Check sheet for the modelled part. Datum: model origin and axes. Units: mm. A direction names the side the tool comes from. Give positions to 0.01 mm unless a question says otherwise; leave off trailing zeros. Order: outer loops, then holes, each group sorted by start corner. A loop starts at its lowest first (then second) coordinate and runs counter-clockwise, first axis right, second up. Notation, with made-up numbers: M -32,50.5 L 2,50.5 A11 cw 2,60.5 Z; hole C 67.25,9.5 d1. An arc over 180 degrees is marked long. Answer in a Markdown table with one row per item. Add a question column.
Autodesk Inventor part; units mm, degrees
ref_plane "YZ Plane" through (0, 0, 0) normal (1, 0, 0) x (0, 1, 0)
ref_plane "XZ Plane" through (0, 0, 0) normal (0, 1, 0) x (-1, 0, 0)
ref_plane "XY Plane" through (0, 0, 0) normal (0, 0, 1) x (1, 0, 0)
sketch "Sketch1" plane through (0, 0, 0) normal (0, 1, 0) x (-1, 0, 0)
  circle A0 centre (0, 0) radius 22.5
  circle A1 centre (0, 0) radius 19
  dimension "d0" = 45
  dimension "d1" = 38
extrude "Extrusion1" add sketch "Sketch1" along normal blind 10
sketch "Sketch2" plane through (0, 10, 0) normal (0, 1, 0) x (1, 0, 0)
  circle A0 centre (0, 0) radius 22.5
  line L0 (0, -22.5) -> (0, 22.5) construction
  circle A1 centre (0, 0) radius 19
  line L1 (-19, 0) -> (19, 0) construction
sketch "Sketch3" plane through (0, 10, 0) normal (0, 1, 0) x (1, 0, 0)
  line L0 (-8, -20) -> (8, -20)
  line L1 (8, -20) -> (8, -40)
  line L2 (8, -40) -> (-8, -40)
  line L3 (-8, -40) -> (-8, -20)
  point P0 (0, 0)
  dimension "d4" = 16
  dimension "d5" = 20
  dimension "d6" = 20
  dimension "d7" = 8
extrude "Extrusion2" add sketch "Sketch3" against normal blind 3
pattern_circular "Circular Pattern1" count 2 over 360 about axis through (0, 0, 0) along (0, 1, 0) of "Extrusion2"
sketch "Sketch4" plane through (0, 10, 0) normal (0, 1, 0) x (1, 0, 0)
  point P0 (0, 0)
sketch "Sketch6" plane through (0, 10, 0) normal (0, 1, 0) x (1, 0, 0)
  line L0 (-20, 5) -> (-38, 5)
  line L1 (-38, 5) -> (-38, 2)
  line L2 (-38, 2) -> (-20, 2)
  line L3 (-20, 2) -> (-20, 5)
  point P0 (0, 0)
  dimension "d14" = 18
  dimension "d15" = 3
  dimension "d16" = 20
  dimension "d17" = 2
extrude "Extrusion3" add sketch "Sketch6" against normal blind 10
pattern_linear "Rectangular Pattern1" count 2 spacing 7 along (0, 0, 1) of "Extrusion3"
sketch "Sketch7" plane through (-38, 10, 2) normal (-1, 0, 0) x (0, 0, 1)
  line L0 (0, 0) -> (0, -10)
  line L1 (-4, 0) -> (-4, -10)
  line L2 (0, -10) -> (-4, -10)
  line L3 (-4, -10) -> (-4, 0)
  line L4 (-4, 0) -> (0, 0)
  line L5 (0, 0) -> (0, -10)
  point P0 (-2, -10)
extrude "Extrusion4" cut sketch "Sketch7" against normal blind 20
sketch "Sketch9" plane through (0, 7, 0) normal (0, -1, 0) x (1, 0, 0)
  point P0 (0, 0)
sketch "Sketch10" plane through (0, 7, 0) normal (0, -1, 0) x (1, 0, 0)
  point P0 (0, 0)
sketch "Sketch11" plane through (8, 10, -40) normal (0, 0, -1) x (-1, 0, 0)
  point P0 (8, -10)
sketch "Sketch13" plane through (-8, 10, -40) normal (-1, 0, 0) x (0, 0, 1)
  point P0 (40, -10)
sketch "Sketch14" plane through (-38, 10, 5) normal (0, 0, 1) x (1, 0, 0)
  circle A0 centre (8, -5) radius 3.25
  line L0 (0, 0) -> (0, -10)
  line L1 (16.0626, -10) -> (0, -10)
  point P0 (38, -10)
  dimension "d27" = 6.5
  dimension "d28" = 8
  dimension "d29" = 5
extrude "Extrusion5" cut sketch "Sketch14" against normal blind 20
sketch "Sketch17" plane through (0, 0, 0) normal (0, -1, 0) x (1, 0, 0)
  arc A0 (-21.9374, -5) -> (-8, -21.0297) centre (0, 0) ccw
  line L0 (-8, -21.0297) -> (-8, -17.2337) construction
  arc A1 (-18.8944, -2) -> (-18.8944, 2) centre (0, 0) ccw
sketch "Sketch21" plane through (-8, 10, -40) normal (-1, 0, 0) x (0, 0, 1)
  line L0 (0, -43) -> (18, -10) construction
  line L1 (62.5, -10) -> (17.5, -10)
  line L2 (18.9703, -3) -> (0, -3)
  line L3 (0, 0) -> (0, -3)
  circle A0 centre (0, -43) radius 40
  line L4 (18.9703, -3) -> (18.9703, -10)
  point P0 (40, -10)
  point P1 (45, -10)
  point P2 (35, -10)
  point P3 (18.9703, -7.7845)
  dimension "d33" = 40
  dimension "d34" = 0
  dimension "d35" = 18
extrude "Extrusion6" add sketch "Sketch21" against normal blind 16 contours A0 L2 L4
sketch "Sketch22" plane through (0, 10, 0) normal (0, 1, 0) x (1, 0, 0)
  circle A0 centre (0, 32) radius 3.25
  line L0 (8, 40) -> (-8, 40)
  point P0 (0, 0)
  dimension "d38" = 6.5
  dimension "d39" = 8
extrude "Extrusion7" cut sketch "Sketch22" against normal blind 16
pattern_circular "Circular Pattern2" count 2 over 360 about axis through (0, 0, 0) along (0, 1, 0) of "Extrusion7", "Extrusion6"
properties part number "motor holder" material "ABS Plastic"
Q1. Draft check along Z on faces 5 (the cylindrical face through (18.983, 4.93, -0.807)), 6 (the flat face through (-29.9, 8.4, -5)), 7 (the flat face through (-8, 8, -29)). Enter one of: pulls with the +Z half, pulls with the -Z half, needs draft (parallel to the pull), parting line crosses it, or undercut.
Q2. Go/stop test with flat-tipped pins: pin 1 (3 mm diameter, centred on x = -33, y = 5.5, fed in from -Z); pin 2 (2.5 mm diameter, centred on y = 6.5, z = 31.5, fed in from -X); pin 3 (2.5 mm diameter, centred on y = 5, z = 29, fed in from +X). Record where each tip stops, or that it passes through.
Q3. Tool access check on faces 1 (the flat face through (-26, 5, -2)), 2 (the cylindrical face through (-26.9, 5.98, -3.48)), 3 (the flat face through (8, 8, 29)), 4 (the flat face through (-30.1, 8.4, 5)). Record the directions out of +Z, -Z, +X, -X, +Y, -Y that give a thin tool (end or side, any length) a straight path to the whole face; none if there is none.
Q4. Cross-section at B-B (y = 3.25). Record the boundary of the cut face in (x, z).
Q5. Cross-section at D-D (x = -9). Record the boundary of the cut face in (y, z).
Q6. Thickness scan on probe 1 along Z at (x, y) = (0, 8.1); probe 2 along Z at (x, y) = (-23, 6); probe 3 along Y at (x, z) = (-30, -4.05). Record the ranges inside material, lowest first.
Q7. Cross-section at C-C (z = 12). Record the boundary of the cut face in (x, y), and give its area (3 significant figures).
Q8. Cross-section at A-A (x = -30). Record the boundary of the cut face in (y, z), and give its area (3 significant figures).
Values follow:
| question | item | result |
|---|---|---|
| 1 | face 5 | undercut |
| 1 | face 6 | pulls with the -Z half |
| 1 | face 7 | needs draft |
| 2 | pin 1 | z = -5 |
| 2 | pin 2 | x = -8 |
| 2 | pin 3 | x = 8 |
| 3 | face 1 | -X, +Y, -Y |
| 3 | face 2 | +Z, -Z |
| 3 | face 3 | +Z, +X, +Y, -Y |
| 3 | face 4 | +Z, -X, +Y, -Y |
| 4 | outline | M -38,-5 L -32.74,-5 L -32.74,-2 L -38,-2 Z; M -38,2 L -32.74,2 L -32.74,5 L -38,5 Z; M -27.26,-5 L -21.94,-5 A22.5 ccw -8,-21.03 L -8,-23.09 L 8,-23.09 L 8,-21.03 A22.5 ccw 8,21.03 L 8,23.09 L -8,23.09 L -8,21.03 A22.5 ccw -21.94,5 L -27.26,5 L -27.26,2 L -18.89,2 A19 cw long -18.89,-2 L -27.26,-2 Z |
| 5 | outline | M 0,-20.62 L 10,-20.62 L 10,-16.73 L 0,-16.73 Z; M 0,16.73 L 10,16.73 L 10,20.62 L 0,20.62 Z |
| 6 | probe 1 | -40 to -35.25, -28.75 to -19, 19 to 28.75, 35.25 to 40 |
| 6 | probe 2 | -5 to -2, 2 to 5 |
| 6 | probe 3 | 0 to 1.75, 8.25 to 10 |
| 7 | outline | M -19.03,0 L -14.73,0 L -14.73,10 L -19.03,10 Z; M 14.73,0 L 19.03,0 L 19.03,10 L 14.73,10 Z |
| 7 | area | 86.0 mm² |
| 8 | outline | M 0,-5 L 1.75,-5 L 1.75,-2 L 0,-2 Z; M 0,2 L 1.75,2 L 1.75,5 L 0,5 Z; M 8.25,-5 L 10,-5 L 10,-2 L 8.25,-2 Z; M 8.25,2 L 10,2 L 10,5 L 8.25,5 Z |
| 8 | area | 21.0 mm² |
